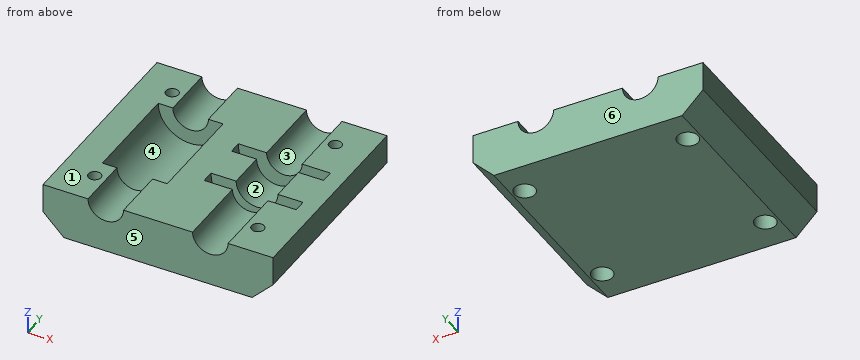
```python
from build123d import *

# Parameters (mm, degrees)
ESQUISSE1_W                  = 55
ESQUISSE1_H                  = 50
BOSS_EXTRU_1_DEPTH           = 12
ESQUISSE2_R                  = 4.25
ENL_V_MAT_EXTRU_1_DEPTH      = 59.311662641
ENL_V_MAT_EXTRU_2_DEPTH      = 12.25
ENL_V_MAT_EXTRU_2_DEPTH_BACK = 12.25
ESQUISSE3_R                  = 7.75
ESQUISSE4_R                  = 11
ENL_V_MAT_EXTRU_3_DEPTH      = 3
ESQUISSE5_R                  = 5
ENL_V_MAT_EXTRU_4_DEPTH      = 15
ENL_V_MAT_EXTRU_5_DEPTH      = 40.05444917
ENL_V_MAT_EXTRU_5_DEPTH_BACK = 40.05444917
ESQUISSE6_R                  = 1.5
ESQUISSE7_R                  = 2.5
ENL_V_MAT_EXTRU_6_DEPTH      = 4
CHANFREIN3_SIZE              = 5


with BuildPart() as part:
    # Esquisse1 → Boss.-Extru.1 (new body)
    with BuildSketch(Plane.XY):
        Rectangle(ESQUISSE1_W, ESQUISSE1_H)
    extrude(amount=BOSS_EXTRU_1_DEPTH)

    # Esquisse2 → Enlèv. mat.-Extru.1 (cut, through all)
    with BuildSketch(Plane(origin=(0, 25, 0), x_dir=(1, 0, 0), z_dir=(0, 1, 0))):
        with Locations((-12.5, -12)):
            Circle(ESQUISSE2_R)
        with Locations((12.5, -12)):
            Circle(ESQUISSE2_R)
    extrude(amount=-ENL_V_MAT_EXTRU_1_DEPTH, mode=Mode.SUBTRACT)

    # Esquisse3 → Enlèv. mat.-Extru.2 (cut, two sides: drawn at the far end of the back side and taken through both)
    with BuildSketch(Plane(origin=(0, 0, 0), x_dir=(1, 0, 0), z_dir=(0, 1, 0)).offset(-ENL_V_MAT_EXTRU_2_DEPTH_BACK)):
        with Locations((-12.5, -12)):
            Circle(ESQUISSE3_R)
    extrude(amount=ENL_V_MAT_EXTRU_2_DEPTH + ENL_V_MAT_EXTRU_2_DEPTH_BACK, mode=Mode.SUBTRACT)

    # Esquisse4 → Enlèv. mat.-Extru.3 (cut)
    with BuildSketch(Plane(origin=(0, 7.5, 0), x_dir=(1, 0, 0), z_dir=(0, 1, 0))):
        with Locations((12.5, -12)):
            Circle(ESQUISSE4_R)
    enl_v_mat_extru_3 = extrude(amount=-ENL_V_MAT_EXTRU_3_DEPTH, mode=Mode.SUBTRACT)

    # Esquisse5 → Enlèv. mat.-Extru.4 (cut)
    with BuildSketch(Plane(origin=(0, 7.5, 0), x_dir=(1, 0, 0), z_dir=(0, 1, 0))):
        with Locations((12.5, -12)):
            Circle(ESQUISSE5_R)
    extrude(amount=-ENL_V_MAT_EXTRU_4_DEPTH, mode=Mode.SUBTRACT)

    # Esquisse6 → Enlèv. mat.-Extru.5 (cut, two sides: drawn at the far end of the back side and taken through both)
    with BuildSketch(Plane(origin=(0, 0, 0), x_dir=(-1, 0, 0), z_dir=(0, 0, -1)).offset(-ENL_V_MAT_EXTRU_5_DEPTH_BACK)):
        with Locations((19.5, -17)):
            Circle(ESQUISSE6_R)
        with Locations((-19.5, -17)):
            Circle(ESQUISSE6_R)
        with Locations((-19.5, 17)):
            Circle(ESQUISSE6_R)
        with Locations((19.5, 17)):
            Circle(ESQUISSE6_R)
    extrude(amount=ENL_V_MAT_EXTRU_5_DEPTH + ENL_V_MAT_EXTRU_5_DEPTH_BACK, mode=Mode.SUBTRACT)

    # Esquisse7 → Enlèv. mat.-Extru.6 (cut)
    with BuildSketch(Plane(origin=(0, 0, 0), x_dir=(-1, 0, 0), z_dir=(0, 0, -1))):
        with Locations((19.5, -17)):
            Circle(ESQUISSE7_R)
        with Locations(Location((19.5, 17, 0), (0, 0, 180))):
            Circle(ESQUISSE7_R)
        with Locations((-19.5, 17)):
            Circle(ESQUISSE7_R)
        with Locations(Location((-19.5, -17, 0), (0, 0, 180))):
            Circle(ESQUISSE7_R)
    extrude(amount=-ENL_V_MAT_EXTRU_6_DEPTH, mode=Mode.SUBTRACT)

    # Chanfrein3
    chanfrein3_edges = [part.edges().sort_by_distance(p)[0] for p in [
        (-27.5, 0, 0),
        (27.5, 0, 0),
    ]]
    chamfer(chanfrein3_edges, length=CHANFREIN3_SIZE)

    # Symétrie2: Enlèv. mat.-Extru.3 across plane
    add(enl_v_mat_extru_3.mirror(Plane.ZX), mode=Mode.SUBTRACT)


solid = part.part
```
Could you check a few things on this model? Use its own coordinates, in mm. Face numbers are marked on the shaded views. A direction names the side the tool comes from. Give positions to 0.01 mm unless a question says otherwise; leave off trailing zeros. Write each loop counter-clockwise with the first axis right and the second up, starting at its lowest first coordinate (ties: lowest second). Pieces come first, ordered by that corner, then holes. Notation, with made-up numbers: (-16.5, -37) - (-0.5, -37) arc R20 cw to (-0.5, -26) - close; hole circle Ø7 at (-8, 2.5). An arc over 180 degrees is marked (long way). One line per item, written item: value. Start each with the question number.
Item 1: Please list where these lines run through material, in increasing order: line 1 (Y direction, x = 19.5, z = 8.5); line 2 (Y direction, x = -19.5, z = 1.7); line 3 (X direction, y = 12, z = 11.75). Write a range as from..to.
Item 2: If we mould it in two halves opening along Y, with no side actions, what happens to the marked faces 3, 4, 5 and 6? For each: +Y half, -Y half, draft (parallel to the pull), parting line (faces both ways), or undercut.
Item 3: Imagine slicing it at A-A, the plane y = -17. List the corners of the cut face in (x, z) for me.
Item 4: Imagine slicing it at C-C, the plane x = -19.5. List the corners of the cut face in (y, z) for me, and give its area (3 significant figures).
Item 5: Imagine slicing it at B-B, the plane x = -12.5. List the corners of the cut face in (y, z) for me.
Item 6: I'm going to push a flat-ended pin straight in: pin 1 (1.5 mm diameter, centred on x = 20, y = -18, fed in from -Z). Where does the tip first touch, or does it pass through?
Item 7: Imagine slicing it at D-D, the plane y = -11.5. List the corners of the cut face in (x, z) for me, and give its area (3 significant figures).
Item 8: Which directions (+Z, -Z, +X, -X, +Y, -Y) give clear straight access to the entire face, cutting with the end or side of a thin tool? Please do the marked faces 1 and 2.
Geometry says:
1. line 1: -25..-18.5, -15.5..-7.5, -4.5..4.5, 7.5..15.5, 18.5..25
1. line 2: -25..-19.5, -14.5..14.5, 19.5..25
1. line 3: -27.5..-20.25, -4.75..8.26, 16.74..27.5
2. face 3: draft
2. face 4: undercut
2. face 5: -Y half
2. face 6: +Y half
3. outline: (-27.5, 5) - (-22.5, 0) - (-22, 0) - (-22, 4) - (-21, 4) - (-21, 12) - (-27.5, 12) - close; (-18, 4) - (-17, 4) - (-17, 0) - (17, 0) - (17, 4) - (18, 4) - (18, 12) - (16.75, 12) arc R4.25 cw to (8.25, 12) - (-8.25, 12) arc R4.25 cw to (-16.75, 12) - (-18, 12) - close; (21, 4) - (22, 4) - (22, 0) - (22.5, 0) - (27.5, 5) - (27.5, 12) - (21, 12) - close
4. outline: (-25, 0) - (-19.5, 0) - (-19.5, 4) - (-18.5, 4) - (-18.5, 12) - (-25, 12) - close; (-15.5, 4) - (-14.5, 4) - (-14.5, 0) - (14.5, 0) - (14.5, 4) - (15.5, 4) - (15.5, 12) - (12.25, 12) - (12.25, 8.67) - (-12.25, 8.67) - (-12.25, 12) - (-15.5, 12) - close; (18.5, 4) - (19.5, 4) - (19.5, 0) - (25, 0) - (25, 12) - (18.5, 12) - close
4. area: 431 mm^2
5. outline: (-25, 0) - (25, 0) - (25, 7.75) - (12.25, 7.75) - (12.25, 4.25) - (-12.25, 4.25) - (-12.25, 7.75) - (-25, 7.75) - close
6. pin 1: z = 4
7. outline: (-27.5, 5) - (-22.5, 0) - (22.5, 0) - (27.5, 5) - (27.5, 12) - (16.75, 12) arc R4.25 cw to (8.25, 12) - (-4.75, 12) arc R7.75 cw to (-20.25, 12) - (-27.5, 12) - close
7. area: 512 mm^2
8. face 1: +Z, +X, -X, +Y, -Y
8. face 2: +Z
